Read the model definition and answer for the solid it produces. Units are mm, in the model's axes. Coordinates: 2 decimals unless noted, no trailing zeros. Order: outer loops, then holes, each group sorted by start corner. A loop starts at its lowest first (then second) coordinate and runs counter-clockwise, first axis right, second up. Notation, with made-up numbers: (84, 38) - (106, 38) arc R11 cw to (106, 52) - close; hole circle Ø11 at (1, 68). An arc over 180 degrees is marked (long way). Use one line per item in the form item = value.
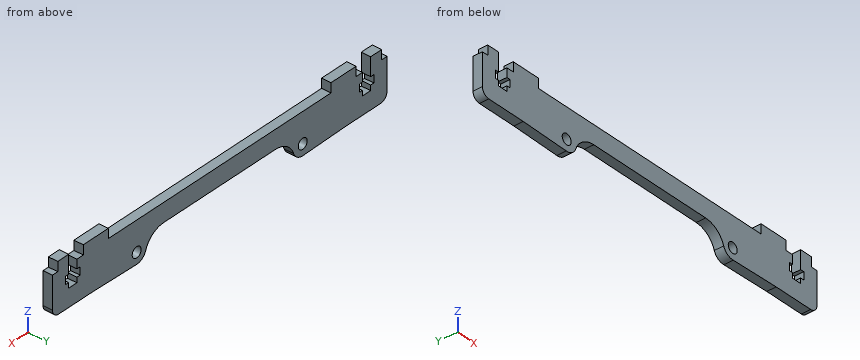
```python
from build123d import *

# Parameters (mm, degrees)
SKETCH1_W           = 9.8
SKETCH1_H           = 3.175
SKETCH1_R           = 3.75
SKETCH1_R_2         = 1.75
SKETCH1_W_2         = 4.3
BOSS_EXTRUDE1_DEPTH = 3.175
FILLET1_DEPTH       = 3.175
FILLET2_R           = 2.5


with BuildPart() as part:
    # Sketch1 → Boss-Extrude1 (new body)
    # profile 1 of 9: a face of its own
    with BuildSketch(Plane(origin=(0, 0, 0), x_dir=(1, 0, 0), z_dir=(0, 1, 0))):
        with BuildLine():
            ThreePointArc((36.25, 0), (32.5, -3.75), (28.75, 0))
            Line((28.75, 0), (28.75, -3.75))
            Line((28.75, -3.75), (-28.75, -3.75))
            Line((-28.75, -3.75), (-28.75, 0))
            ThreePointArc((-28.75, 0), (-32.5, -3.75), (-36.25, 0))
            Line((-36.25, 0), (-36.25, -3.75))
            Line((-36.25, -3.75), (-49.5, -3.75))
            Line((-49.5, -3.75), (-49.5, 3.325))
            Line((-49.5, 3.325), (-65.5, 3.325))
            Line((-65.5, 3.325), (-65.5, -10))
            Line((-65.5, -10), (-63.4, -10))
            Line((-63.4, -10), (-59.1, -10))
            Line((-59.1, -10), (-59.1, -7))
            Line((-59.1, -7), (-60.35, -7))
            Line((-60.35, -7), (-60.35, -4.4))
            Line((-60.35, -4.4), (-59.1, -4.4))
            Line((-59.1, -4.4), (-59.1, -2.675))
            Line((-59.1, -2.675), (-55.9, -2.675))
            Line((-55.9, -2.675), (-55.9, -4.4))
            Line((-55.9, -4.4), (-54.65, -4.4))
            Line((-54.65, -4.4), (-54.65, -7))
            Line((-54.65, -7), (-55.9, -7))
            Line((-55.9, -7), (-55.9, -10))
            Line((-55.9, -10), (-53.4, -10))
            Line((-53.4, -10), (-43.6, -10))
            Line((-43.6, -10), (43.6, -10))
            Line((43.6, -10), (53.4, -10))
            Line((53.4, -10), (55.9, -10))
            Line((55.9, -10), (55.9, -7))
            Line((55.9, -7), (54.65, -7))
            Line((54.65, -7), (54.65, -4.4))
            Line((54.65, -4.4), (55.9, -4.4))
            Line((55.9, -4.4), (55.9, -2.675))
            Line((55.9, -2.675), (59.1, -2.675))
            Line((59.1, -2.675), (59.1, -4.4))
            Line((59.1, -4.4), (60.35, -4.4))
            Line((60.35, -4.4), (60.35, -7))
            Line((60.35, -7), (59.1, -7))
            Line((59.1, -7), (59.1, -10))
            Line((59.1, -10), (63.4, -10))
            Line((63.4, -10), (65.5, -10))
            Line((65.5, -10), (65.5, 3.325))
            Line((65.5, 3.325), (49.5, 3.325))
            Line((49.5, 3.325), (49.5, -3.75))
            Line((49.5, -3.75), (36.25, -3.75))
            Line((36.25, -3.75), (36.25, 0))
        make_face()
    # profile 2 of 9: a face of its own
    with BuildSketch(Plane(origin=(0, 0, 0), x_dir=(1, 0, 0), z_dir=(0, 1, 0))):
        with Locations((-48.5, -11.5875)):
            Rectangle(SKETCH1_W, SKETCH1_H)
    # profile 3 of 9: a face of its own
    with BuildSketch(Plane(origin=(0, 0, 0), x_dir=(1, 0, 0), z_dir=(0, 1, 0))):
        with Locations((-32.5, 0)):
            Circle(SKETCH1_R)
        with Locations(Location((-32.5, 0, 0), (0, 0, 270))):
            Circle(SKETCH1_R_2, mode=Mode.SUBTRACT)
    # profile 4 of 9: a face of its own
    with BuildSketch(Plane(origin=(0, 0, 0), x_dir=(1, 0, 0), z_dir=(0, 1, 0))):
        with Locations((32.5, 0)):
            Circle(SKETCH1_R)
        with Locations(Location((32.5, 0, 0), (0, 0, 270))):
            Circle(SKETCH1_R_2, mode=Mode.SUBTRACT)
    # profile 5 of 9: a face of its own
    with BuildSketch(Plane(origin=(0, 0, 0), x_dir=(1, 0, 0), z_dir=(0, 1, 0))):
        with Locations((48.5, -11.5875)):
            Rectangle(SKETCH1_W, SKETCH1_H)
    # profile 6 of 9: a face of its own
    with BuildSketch(Plane(origin=(0, 0, 0), x_dir=(1, 0, 0), z_dir=(0, 1, 0))):
        with Locations((-61.25, -11.5875)):
            Rectangle(SKETCH1_W_2, SKETCH1_H)
    # profile 7 of 9: a face of its own
    with BuildSketch(Plane(origin=(0, 0, 0), x_dir=(1, 0, 0), z_dir=(0, 1, 0))):
        with Locations((61.25, -11.5875)):
            Rectangle(SKETCH1_W_2, SKETCH1_H)
    # profile 8 of 9: a face of its own
    with BuildSketch(Plane(origin=(0, 0, 0), x_dir=(1, 0, 0), z_dir=(0, 1, 0))):
        with BuildLine():
            Line((-36.25, -3.75), (-36.25, 0))
            ThreePointArc((-36.25, 0), (-35.217092731, 2.584551622), (-32.687382886, 3.745315428))
            Line((-32.687382886, 3.745315428), (-49.5, 3.325))
            Line((-49.5, 3.325), (-49.5, -3.75))
            Line((-49.5, -3.75), (-36.25, -3.75))
        make_face()
    # profile 9 of 9: a face of its own
    with BuildSketch(Plane(origin=(0, 0, 0), x_dir=(1, 0, 0), z_dir=(0, 1, 0))):
        with BuildLine():
            ThreePointArc((32.687382886, 3.745315428), (35.217092731, 2.584551622), (36.25, 0))
            Line((36.25, 0), (36.25, -3.75))
            Line((36.25, -3.75), (49.5, -3.75))
            Line((49.5, -3.75), (49.5, 3.325))
            Line((49.5, 3.325), (32.687382886, 3.745315428))
        make_face()
    extrude(amount=BOSS_EXTRUDE1_DEPTH)

    # Fillet1: read off the stored shape, not the designer's step
    # Fillet1 outline → Fillet1 (add)
    with BuildSketch(Plane(origin=(0, 0, 0), x_dir=(1, 0, 0), z_dir=(0, 1, 0))):
        with BuildLine():
            Line((-28.75, -3.75), (-21.893398282, -3.75))
            ThreePointArc((-21.893398282, -3.75), (-26.223525301, -2.373724357), (-28.964466094, 1.25))
            ThreePointArc((-28.964466094, 1.25), (-28.804005402, 0.63413242), (-28.75, 0))
            Line((-28.75, 0), (-28.75, -3.75))
        make_face()
        with BuildLine():
            ThreePointArc((28.964466094, 1.25), (26.223525301, -2.373724357), (21.893398282, -3.75))
            Line((21.893398282, -3.75), (28.75, -3.75))
            Line((28.75, -3.75), (28.75, 0))
            ThreePointArc((28.75, 0), (28.804005402, 0.63413242), (28.964466094, 1.25))
        make_face()
    extrude(amount=FILLET1_DEPTH)

    # Fillet2
    fillet2_edges = [part.edges().sort_by_distance(p)[0] for p in [
        (65.5, 1.5875, -3.325),
        (-65.5, 1.5875, -3.325),
    ]]
    fillet(fillet2_edges, radius=FILLET2_R)


solid = part.part
```
(1) Section C-C, the plane x = 17.5 is taken. Write down the section's boundary in (y, z) (3 decimals).
Answer list:
outline = (0, 3.75) - (3.175, 3.75) - (3.175, 10) - (0, 10) - close
(2) Section B-B, the plane z = 5.75 is taken. Write down the section's boundary in (x, y) (3 decimals), then the cut area to 3 significant figures.
Answer list:
outline = (-65.5, 0) - (-60.35, 0) - (-60.35, 3.175) - (-65.5, 3.175) - close; (-54.65, 0) - (54.65, 0) - (54.65, 3.175) - (-54.65, 3.175) - close; (60.35, 0) - (65.5, 0) - (65.5, 3.175) - (60.35, 3.175) - close
area = 380 mm2
(3) Section A-A, the plane z = 11.25 is taken. Write down the section's boundary in (x, y) (3 decimals).
Answer list:
outline = (-63.4, 0) - (-59.1, 0) - (-59.1, 3.175) - (-63.4, 3.175) - close; (-53.4, 0) - (-43.6, 0) - (-43.6, 3.175) - (-53.4, 3.175) - close; (43.6, 0) - (53.4, 0) - (53.4, 3.175) - (43.6, 3.175) - close; (59.1, 0) - (63.4, 0) - (63.4, 3.175) - (59.1, 3.175) - close
(4) Section D-D, the plane y = 2.25 is taken. State how many separate pieces and enclosed holes the cut face has, then the cut area to 3 significant figures.
Answer list:
separate_pieces = 1
enclosed_holes = 2
area = 1,370 mm2
(5) Given pin 1 Ø0.8 at (x, y) = (-54.5, 2.5) entering from +Z; pin 2 Ø4 at (x, z) = (32.5, 0) entering from -Y; pin 3 Ø1 at (y, z) = (1, 12) entering from +X; pin 4 Ø0.6 at (x, y) = (60, 2.5) entering from -Z (3 decimals), each flat-ended and moving along its own axis, determine where each tip first touches the part or whether it passes through.
Answer list:
pin_1 = 10
pin_2 = 0
pin_3 = 63.4
pin_4 = -3.325
(6) Straight lines are drawn through the part: L1, parallel to X at y = 1.2, z = 8; L2, parallel to X at y = 2.05, z = 10.75; L3, parallel to X at y = 0.65, z = 5.5. For each, find the intervals that lie inside material, in ascending order.
Answer list:
L1 = -65.5 to -59.1, -55.9 to 55.9, 59.1 to 65.5
L2 = -63.4 to -59.1, -53.4 to -43.6, 43.6 to 53.4, 59.1 to 63.4
L3 = -65.5 to -60.35, -54.65 to 54.65, 60.35 to 65.5
